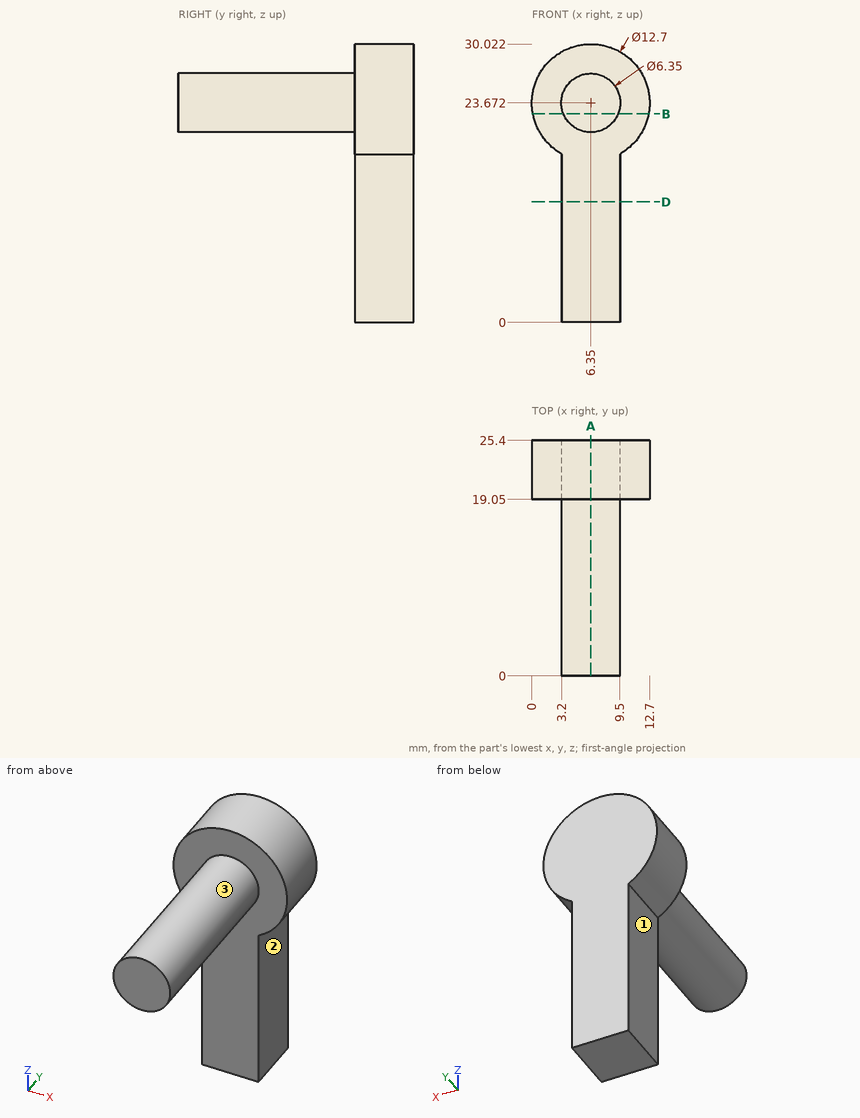
Input: dimensioned drawing with shaded views. Units: mm. Origin: part minimum x, y, z. A direction names the side the tool comes from. Coordinates: 2 decimals unless noted, no trailing zeros. Write each loop counter-clockwise with the first axis right and the second up, starting at its lowest first coordinate (ties: lowest second). Pieces come first, ordered by that corner, then holes. Notation, with made-up numbers: M 13.5,-5.5 L 38.5,-5.5 A26 ccw 38.5,12.5 Z; hole C 83,40 d4. An arc over 180 degrees is marked long. Use a Markdown table: item, result.
1) Section D-D, the plane z = 13. Output: boundary loops of the cut face in (x, y), then the cut area to 3 significant figures.
Conclusion:
| item | result |
|---|---|
| outline | M 3.2,19.05 L 9.5,19.05 L 9.5,25.4 L 3.2,25.4 Z |
| area | 40.0 mm^2 |
2) Section A-A, the plane x = 6.35. Output: boundary loops of the cut face in (y, z).
Conclusion:
| item | result |
|---|---|
| outline | M 0,20.5 L 19.05,20.5 L 19.05,0 L 25.4,0 L 25.4,30.02 L 19.05,30.02 L 19.05,26.85 L 0,26.85 Z |
3) Section B-B, the plane z = 22.5. Output: boundary loops of the cut face in (x, y), then the cut area to 3 significant figures.
Conclusion:
| item | result |
|---|---|
| outline | M 0.11,19.05 L 3.4,19.05 L 3.4,0 L 9.3,0 L 9.3,19.05 L 12.59,19.05 L 12.59,25.4 L 0.11,25.4 Z |
| area | 192 mm^2 |
4) Reachability of the marked faces 1, 2 and 3 from +Z, -Z, +X, -X, +Y, -Y: full face, straight path, thin tool, end or side. Return the list, or none.
Conclusion:
| item | result |
|---|---|
| face 1 | -Z, -X, +Y, -Y |
| face 2 | -Z, +X, +Y, -Y |
| face 3 | -Y |
5) First-contact query: pin 1 Ø5 at (y, z) = (22.5, 6.5) entering from -X; pin 2 Ø10 at (y, z) = (4, 11) entering from -X; pin 3 Ø5 at (y, z) = (17.5, 3) entering from +X; pin 4 Ø4 at (x, y) = (7.5, 4.5) entering from +Z. Flat tips, straight axial feed; report the tip coordinate or a pass-through.
Conclusion:
| item | result |
|---|---|
| pin 1 | stops at x = 3.2 |
| pin 2 | passes through |
| pin 3 | stops at x = 9.5 |
| pin 4 | stops at z = 26.85 |
6) Ray query, L1, parallel to Y at x = 9.5, z = 28.5; L2, parallel to X at y = 23.75, z = 12; L3, parallel to Z at x = 4, y = 7. Return the intervals inside material, ascending.
Conclusion:
| item | result |
|---|---|
| L1 | y = 19.05 to 25.4 |
| L2 | x = 3.2 to 9.5 |
| L3 | z = 21.54 to 25.81 |
